Geometry: final body of the model. Coordinates: model frame, mm. A direction names the side the tool comes from. Give positions to 0.01 mm unless a question says otherwise; leave off trailing zeros. Loops run counter-clockwise (first coordinate to the right, second up) from the corner with the lowest first, then second, coordinate; pieces in that order, holes last. Notation, with made-up numbers: (49.5, 11) -> (98.5, 11) arc R26 ccw to (98.5, 28) -> close; hole circle Ø10 at (43.5, 85.25). An arc over 180 degrees is marked (long way). One line per question, with ' | ' between items. Start each with the question number.
Item 1: Section C-C on y = 10. Return loops of the section in (x, z), then the cut area to 3 significant figures.
Item 2: Pin query (flat end, axial travel): P1, Ø1.5, axis at x = 0, y = 10, coming from the -Z side; P2, Ø3, axis at y = 10, z = 19.5, coming from the -X side. Return the tip coordinate at first contact, or that it passes through.
Item 3: Mould query, pull axis Y, two halves, no side actions, for faces 3 (the flat face through (2.5, 10, 22)), 4 (the flat face through (0, 20, 15)), 5 (the cylindrical face through (0.75, 11.03, 10.85)). Classes: released by +Y, released by -Y, zero draft, split by the parting line, or undercut.
Item 4: Set-up query: faces 1 (the cylindrical face through (0.035, 19.699, 34.715)), 2 (the flat face through (0, 4, 2)). Return all of +Z, -Z, +X, -X, +Y, -Y with unobstructed straight access to the full face (end or side cutting, diameter ignored); none if empty.
Item 5: Material intervals for line 1 along Y through (x, z) = (1.3, 12.2); line 2 along Y through (x, z) = (1.4, 1); line 3 along Z through (x, y) = (0, 17.05), sorted ascending. Write a range as [from, to].
Item 6: Section B-B on z = 19.5. Return loops of the section in (x, y).
Item 7: Section A-A on x = 0. Return loops of the section in (y, z).
Item 8: Section D-D on z = 2.5. Return loops of the section in (x, y), then the cut area to 3 significant figures.
from build123d import *

# Parameters (mm, degrees)
SKETCHSIDE_R                          = 0.5
BOSSEXTRUDESIDE_DEPTH                 = 20
CUTEXTRUDEDISTALROOM_DEPTH            = 41.388736054
CUTEXTRUDEDISTALROOM_DEPTH_BACK       = 41.388736054
SKETCHDISTALROOM_W                    = 9
SKETCHDISTALROOM_H                    = 12
FILLETBUTTOM_R                        = 1
CSKM3FLATHEADMACHINESCREW_D           = 3.4
CSKM3FLATHEADMACHINESCREW_CSINK_D     = 6.3
CSKM3FLATHEADMACHINESCREW_CSINK_ANGLE = 90


with BuildPart() as part:
    # SketchSide → BossExtrudeSide (new body)
    with BuildSketch(Plane(origin=(0, 0, 0), x_dir=(1, 0, 0), z_dir=(0, 1, 0))):
        with BuildLine():
            Line((-2.5, -35), (2.5, -35))
            Line((2.5, -35), (2.5, 0))
            ThreePointArc((2.5, 0), (0, 2.5), (-2.5, 0))
            Line((-2.5, 0), (-2.5, -35))
        make_face()
        with Locations(Location((0, 0, 0), (0, 0, 270))):
            Circle(SKETCHSIDE_R, mode=Mode.SUBTRACT)
    extrude(amount=BOSSEXTRUDESIDE_DEPTH)

    # SketchDistalRoom → CutExtrudeDistalRoom (cut, two sides: drawn at the far end of the back side and taken through both)
    with BuildSketch(Plane(origin=(0, 0, 0), x_dir=(0, 0, -1), z_dir=(1, 0, 0)).offset(-CUTEXTRUDEDISTALROOM_DEPTH_BACK)):
        with Locations((-2, 10)):
            Rectangle(SKETCHDISTALROOM_W, SKETCHDISTALROOM_H)
    extrude(amount=CUTEXTRUDEDISTALROOM_DEPTH + CUTEXTRUDEDISTALROOM_DEPTH_BACK, mode=Mode.SUBTRACT)

    # FilletButtom
    filletbuttom_edges = [part.edges().sort_by_distance(p)[0] for p in [
        (0, 0, 35),
        (0, 20, 35),
    ]]
    fillet(filletbuttom_edges, radius=FILLETBUTTOM_R)

    # CSKM3FlatHeadMachineScrew (through all)
    with Locations(Plane(origin=(-2.5, 10, 12.2), x_dir=(0, 0, -1), z_dir=(-1, 0, 0))):
        with Locations((0, 0), (-7.3, 0)):
            CounterSinkHole(CSKM3FLATHEADMACHINESCREW_D / 2, CSKM3FLATHEADMACHINESCREW_CSINK_D / 2, counter_sink_angle=CSKM3FLATHEADMACHINESCREW_CSINK_ANGLE)


solid = part.part
Result sheet:
1) outline: (-2.5, 6.5) -> (2.5, 6.5) -> (2.5, 10.5) -> (-1.05, 10.5) -> (-2.5, 9.05) -> close; (-2.5, 15.35) -> (-1.05, 13.9) -> (2.5, 13.9) -> (2.5, 17.8) -> (-1.05, 17.8) -> (-2.5, 16.35) -> close; (-2.5, 22.65) -> (-1.05, 21.2) -> (2.5, 21.2) -> (2.5, 35) -> (-2.5, 35) -> close | area: 104 mm²
2) P1: stops at z = 6.5 | P2: passes through
3) face 3: zero draft | face 4: released by +Y | face 5: undercut
4) face 1: +Z, +X, -X, +Y | face 2: -Z, +X, -X
5) line 1: y = [0, 8.3], [11.7, 20] | line 2: y = [0, 4], [16, 20] | line 3: z = [-2.5, -0.5], [0.5, 35]
6) outline: (-2.5, 0) -> (2.5, 0) -> (2.5, 8.3) -> (-1.05, 8.3) -> (-2.5, 6.85) -> close; (-2.5, 13.15) -> (-1.05, 11.7) -> (2.5, 11.7) -> (2.5, 20) -> (-2.5, 20) -> close
7) outline: (0, -2.5) -> (4, -2.5) -> (4, -0.5) -> (0, -0.5) -> close; (0, 0.5) -> (4, 0.5) -> (4, 6.5) -> (16, 6.5) -> (16, 0.5) -> (20, 0.5) -> (20, 34) arc R1 ccw to (19, 35) -> (1, 35) arc R1 ccw to (0, 34) -> close; (16, -2.5) -> (20, -2.5) -> (20, -0.5) -> (16, -0.5) -> close; hole circle Ø3.4 at (10, 12.2); hole circle Ø3.4 at (10, 19.5)
8) outline: (-2.5, 0) -> (2.5, 0) -> (2.5, 4) -> (-2.5, 4) -> close; (-2.5, 16) -> (2.5, 16) -> (2.5, 20) -> (-2.5, 20) -> close | area: 40.0 mm²
